Can you work these out from the model? Positions are in its coordinate system, mm. Give positions to 0.01 mm unless a question says otherwise; leave off trailing zeros. Loops run counter-clockwise (first coordinate to the right, second up) from the corner with the lowest first, then second, coordinate; pieces in that order, holes last. Notation, with made-up numbers: M 54,23.25 L 60,23.25 A19 ccw 60,48.25 Z; hole C -20.5,15 d4. An arc over 180 degrees is marked long. Use CSV: the item, a comma, the result in double quotes.
Autodesk Inventor part; units mm, degrees
ref_plane "YZ Plane" through (0, 0, 0) normal (1, 0, 0) x (0, 1, 0)
ref_plane "XZ Plane" through (0, 0, 0) normal (0, 1, 0) x (-1, 0, 0)
ref_plane "XY Plane" through (0, 0, 0) normal (0, 0, 1) x (1, 0, 0)
sketch "Sketch1" plane through (0, 0, 0) normal (1, 0, 0) x (0, 1, 0)
  line L0 (21.8571, 39) -> (9.8571, 39)
  line L1 (9.8571, 39) -> (9.8571, -39)
  line L2 (9.8571, -39) -> (21.8571, -39)
  line L3 (21.8571, -39) -> (21.8571, 39)
  line L4 (9.8571, 0) -> (21.8571, 0)
  point P0 (0, 0)
  point P1 (15.8571, 33)
  point P2 (15.8571, -33)
  dimension "d0" = 78
  dimension "d1" = 12
  dimension "d2" = 6
  dimension "d3" = 6
  dimension "d4" = 39
extrude "Extrusion1" add sketch "Sketch1" along normal blind 6
hole "Hole1" at (0, 15.8571, 33) at (0, 15.8571, -33) direction (1, 0, 0) diameter 4.5 end through all
properties part number "Weight Baby"
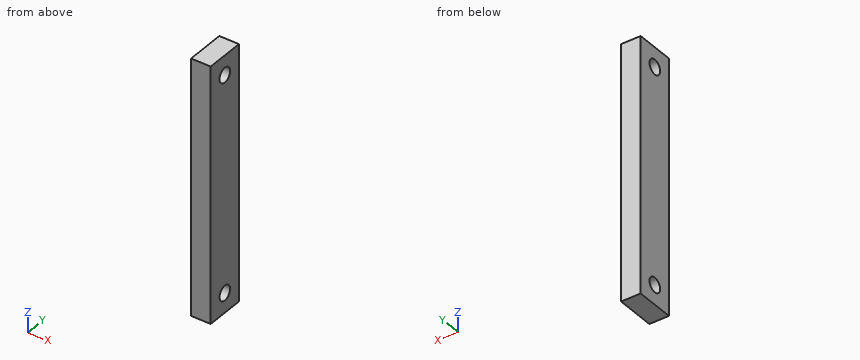
Q1. Please list where these lines run through material, in increasing order: L1, parallel to Y at x = 2.65, z = 33; L2, parallel to Z at x = 1.65, y = 14.5; L3, parallel to Z at x = 4.2, y = 17.5. Write a range as from..to.
Model answer:
L1,"9.86..13.61, 18.11..21.86"
L2,"-39..-34.79, -31.21..31.21, 34.79..39"
L3,"-39..-34.54, -31.46..31.46, 34.54..39"
Q2. I want a section at C-C, the plane x = 2.55. Please give me the cut outline in (y, z).
Model answer:
outline,"M 9.86,-39 L 21.86,-39 L 21.86,39 L 9.86,39 Z; hole C 15.86,-33 d4.5; hole C 15.86,33 d4.5"
Q3. I want a section at A-A, the plane z = 33. Please give me the cut outline in (x, y).
Model answer:
outline,"M 0,9.86 L 6,9.86 L 6,13.61 L 0,13.61 Z; M 0,18.11 L 6,18.11 L 6,21.86 L 0,21.86 Z"
Q4. I want a section at B-B, the plane y = 16.75. Please give me the cut outline in (x, z).
Model answer:
outline,"M 0,-39 L 6,-39 L 6,-35.07 L 0,-35.07 Z; M 0,-30.93 L 6,-30.93 L 6,30.93 L 0,30.93 Z; M 0,35.07 L 6,35.07 L 6,39 L 0,39 Z"
Q5. I'm going to push a flat-ended pin straight in: P1, Ø6, axis at y = 15.86, z = 33, coming from the +X side. Where does the tip first touch, or does it pass through?
Model answer:
P1,"x = 6"
